Geometry check sheet. Reference: the model listing, model coordinates, mm. Round coordinates to 2 decimals unless told otherwise and drop trailing zeros. Loops run counter-clockwise (first coordinate to the right, second up) from the corner with the lowest first, then second, coordinate; pieces in that order, holes last. Notation, with made-up numbers: (67.25, 25) - (73.25, 25) arc R13 cw to (73.25, 40) - close; hole circle Ø2 at (36, -26). An arc over 180 degrees is marked (long way). Write item = value, one per line.
```python
from build123d import *

# Parameters (mm, degrees)
SKETCH1_R           = 6
SKETCH1_R_2         = 1.25
SKETCH1_R_3         = 1.65
SKETCH1_W           = 10
SKETCH1_H           = 3
BOSS_EXTRUDE2_DEPTH = 3


with BuildPart() as part:
    # Sketch1 → Boss-Extrude2 (new body)
    with BuildSketch(Plane.XY):
        Polygon((25, 5), (25, -5.5), (25, -40.5), (5, -40.5), (5, -37.5), (-5, -37.5), (-5, -40.5), (-25, -40.5), (-25, -5.5), (-25, 4.5), (-25, 24.5), (-25, 54.5), (-5, 54.5), (-5, 51.5), (5, 51.5), (5, 54.5), (25, 54.5), (25, 24.5), align=None)
        Circle(SKETCH1_R, mode=Mode.SUBTRACT)
        with Locations((-15.5, 15.5)):
            Circle(SKETCH1_R_2, mode=Mode.SUBTRACT)
        with Locations((15.5, 15.5)):
            Circle(SKETCH1_R_2, mode=Mode.SUBTRACT)
        with Locations((15.5, -15.5)):
            Circle(SKETCH1_R_2, mode=Mode.SUBTRACT)
        with Locations((-15.5, -15.5)):
            Circle(SKETCH1_R_2, mode=Mode.SUBTRACT)
        with Locations((-17.5, -8)):
            Circle(SKETCH1_R_3, mode=Mode.SUBTRACT)
        with Locations((17.5, -8)):
            Circle(SKETCH1_R_3, mode=Mode.SUBTRACT)
        with Locations((-15, 50)):
            Rectangle(SKETCH1_W, SKETCH1_H, mode=Mode.SUBTRACT)
        with Locations((15, 50)):
            Rectangle(SKETCH1_W, SKETCH1_H, mode=Mode.SUBTRACT)
    extrude(amount=BOSS_EXTRUDE2_DEPTH)


solid = part.part
```
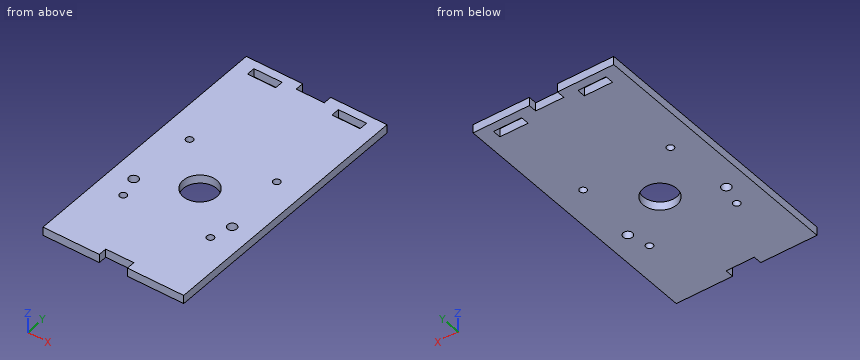
(1) Section check A-A (y = 0). Enter the section's corners in (x, z).
Answers follow:
outline = (-25, 0) - (-6, 0) - (-6, 3) - (-25, 3) - close; (6, 0) - (25, 0) - (25, 3) - (6, 3) - close
(2) Section check B-B (z = 1.65). State how many separate pieces and enclosed holes the cut face has, then the cut area to 3 significant figures.
Answers follow:
separate_pieces = 1
enclosed_holes = 9
area = 4,480 mm²
(3) Section check C-C (x = 11.5). Enter the section's corners in (y, z).
Answers follow:
outline = (-40.5, 0) - (48.5, 0) - (48.5, 3) - (-40.5, 3) - close; (51.5, 0) - (54.5, 0) - (54.5, 3) - (51.5, 3) - close
(4) Scan lines: L1, parallel to Y at x = 15.5, z = 1; L2, parallel to Y at x = 10.5, z = 0.85; L3, parallel to X at y = -9.5, z = 0.85. Record each from-to range of solid material in increasing order. Write a range as [from, to].
Answers follow:
L1 = [-40.5, -16.75], [-14.25, 14.25], [16.75, 48.5], [51.5, 54.5]
L2 = [-40.5, 48.5], [51.5, 54.5]
L3 = [-25, -18.19], [-16.81, 16.81], [18.19, 25]
(5) Section check D-D (y = 15.5). Enter the section's corners in (x, z).
Answers follow:
outline = (-25, 0) - (-16.75, 0) - (-16.75, 3) - (-25, 3) - close; (-14.25, 0) - (14.25, 0) - (14.25, 3) - (-14.25, 3) - close; (16.75, 0) - (25, 0) - (25, 3) - (16.75, 3) - close
(6) Gauge pin test, flat end, axial feed: pin 1 (1 mm diameter, centred on x = -0.5, z = 2.5, fed in from -Y). Record the tip position at first contact, or that the pin passes through.
Answers follow:
pin_1 = -37.5
